Here's how the part is built. I have some questions about the finished solid (model axes, mm). A direction names the side the tool comes from. Coordinates: 2 decimals unless noted, no trailing zeros. Write each loop counter-clockwise with the first axis right and the second up, starting at its lowest first coordinate (ties: lowest second). Pieces come first, ordered by that corner, then holes.
from build123d import *

# Parameters (mm, degrees)
F0_W         = 30
F0_H         = 30
F1_DEPTH     = 30
F2_R         = 5
F3_DEPTH     = 30
F4_R         = 2.5001325449
F5_DEPTH     = 60.001
F6_T1_DEPTH  = 20
F6_T3_DEPTH  = 20
F6_T5_DEPTH  = 20
F6_S9_W      = 5.1
F6_S9_H      = 5.1
F6_T10_DEPTH = 5.1
F6_S15_W     = 5.1
F6_S15_H     = 5.1
F6_T16_DEPTH = 5.1
F6_S21_W     = 5.1
F6_S21_H     = 5.1
F6_T22_DEPTH = 5.1
F6_S27_W     = 5.1
F6_S27_H     = 5.1
F6_T28_DEPTH = 5.1
F6_S33_W     = 5.1
F6_S33_H     = 5.1
F6_T34_DEPTH = 5.1
F6_S39_W     = 5.1
F6_S39_H     = 5.1
F6_T40_DEPTH = 5.1
F6_S45_W     = 5.1
F6_S45_H     = 5.1
F6_T46_DEPTH = 5.1
F6_S51_W     = 5.1
F6_S51_H     = 5.1
F6_T52_DEPTH = 5.1


# Not quite as in the source:
# - a fillet or chamfer that OpenCascade refuses, or shapes differently, is made with other operations: its cross-section is extruded or revolved along the edge and cut away or added


with BuildPart() as f1:
    # F0 (on Front) → F1 (new body)
    with BuildSketch(Plane.XZ):
        Rectangle(F0_W, F0_H)
    extrude(amount=F1_DEPTH)

    # F2 (on face) → F3 (join)
    with BuildSketch(Plane.XZ.offset(30)):
        Circle(F2_R)
    extrude(amount=F3_DEPTH)

    # F4 (on face) → F5 (cut, through all)
    with BuildSketch(Plane.XZ.offset(60)):
        Circle(F4_R)
    extrude(amount=-F5_DEPTH, mode=Mode.SUBTRACT)

    # F6: fillet of radius 5 on 13 edges, made by hand

    # F6_s2 → F6_t1 (cut)
    with BuildSketch(Plane.XZ.offset(5)):
        with BuildLine():
            ThreePointArc((10, 15), (13.5355339059, 13.5355339059), (15, 10))
            Line((15, 10), (15, 15))
            Line((15, 15), (10, 15))
        make_face()
        with BuildLine():
            ThreePointArc((-10, 15), (-13.5355339059, 13.5355339059), (-15, 10))
            Line((-15, 10), (-15, 15))
            Line((-15, 15), (-10, 15))
        make_face()
        with BuildLine():
            ThreePointArc((-15, -10), (-13.5355339059, -13.5355339059), (-10, -15))
            Line((-10, -15), (-15, -15))
            Line((-15, -15), (-15, -10))
        make_face()
        with BuildLine():
            ThreePointArc((15, -10), (13.5355339059, -13.5355339059), (10, -15))
            Line((10, -15), (15, -15))
            Line((15, -15), (15, -10))
        make_face()
    extrude(amount=F6_T1_DEPTH, mode=Mode.SUBTRACT)

    # F6_s4 → F6_t3 (cut)
    with BuildSketch(Plane.YZ.offset(-10)):
        with BuildLine():
            ThreePointArc((-25, 15), (-28.5355339059, 13.5355339059), (-30, 10))
            Line((-30, 10), (-30, 15))
            Line((-30, 15), (-25, 15))
        make_face()
        with BuildLine():
            ThreePointArc((-5, 15), (-1.4644660941, 13.5355339059), (0, 10))
            Line((0, 10), (0, 15))
            Line((0, 15), (-5, 15))
        make_face()
        with BuildLine():
            ThreePointArc((-30, -10), (-28.5355339059, -13.5355339059), (-25, -15))
            Line((-25, -15), (-30, -15))
            Line((-30, -15), (-30, -10))
        make_face()
        with BuildLine():
            ThreePointArc((0, -10), (-1.4644660941, -13.5355339059), (-5, -15))
            Line((-5, -15), (0, -15))
            Line((0, -15), (0, -10))
        make_face()
    extrude(amount=F6_T3_DEPTH, mode=Mode.SUBTRACT)

    # F6_s6 → F6_t5 (cut)
    with BuildSketch(Plane.XY.offset(-10)):
        with BuildLine():
            ThreePointArc((-15, -5), (-13.5355339059, -1.4644660941), (-10, 0))
            Line((-10, 0), (-15, 0))
            Line((-15, 0), (-15, -5))
        make_face()
        with BuildLine():
            ThreePointArc((-15, -25), (-13.5355339059, -28.5355339059), (-10, -30))
            Line((-10, -30), (-15, -30))
            Line((-15, -30), (-15, -25))
        make_face()
        with BuildLine():
            ThreePointArc((15, -5), (13.5355339059, -1.4644660941), (10, 0))
            Line((10, 0), (15, 0))
            Line((15, 0), (15, -5))
        make_face()
        with BuildLine():
            ThreePointArc((15, -25), (13.5355339059, -28.5355339059), (10, -30))
            Line((10, -30), (15, -30))
            Line((15, -30), (15, -25))
        make_face()
    extrude(amount=F6_T5_DEPTH, mode=Mode.SUBTRACT)


with BuildPart() as f6_tool8:
    # F6_s9 → F6_t10 (new body)
    with BuildSketch(Plane.XY.offset(10)):
        with Locations((12.55, -2.45)):
            Rectangle(F6_S9_W, F6_S9_H)
    extrude(amount=F6_T10_DEPTH)

    # F6_s11 → F6_t12 (revolve, cut)
    with BuildSketch(Plane(origin=(10, -5, 10), x_dir=(-0.7071067812, -0.7071067812, 0), z_dir=(-0.7071067812, 0.7071067812, 0))):
        with BuildLine():
            ThreePointArc((0, -5), (5, 0), (0, 5))
            Line((0, 5), (0, -5))
        make_face()
    revolve(axis=Axis((10, -5, 10), (0, 0, 1)), mode=Mode.SUBTRACT)


with BuildPart() as f1_1:
    add(f1.part)

    # F6_t7: cut F6_tool8
    add(f6_tool8.part, mode=Mode.SUBTRACT)


with BuildPart() as f6_tool14:
    # F6_s15 → F6_t16 (new body)
    with BuildSketch(Plane.XY.offset(10)):
        with Locations((12.55, -27.55)):
            Rectangle(F6_S15_W, F6_S15_H)
    extrude(amount=F6_T16_DEPTH)

    # F6_s17 → F6_t18 (revolve, cut)
    with BuildSketch(Plane(origin=(10, -25, 10), x_dir=(-0.7071067812, 0.7071067812, 0), z_dir=(0.7071067812, 0.7071067812, 0))):
        with BuildLine():
            ThreePointArc((0, -5), (5, 0), (0, 5))
            Line((0, 5), (0, -5))
        make_face()
    revolve(axis=Axis((10, -25, 10), (0, 0, 1)), mode=Mode.SUBTRACT)


with BuildPart() as f1_2:
    add(f1_1.part)

    # F6_t13: cut F6_tool14
    add(f6_tool14.part, mode=Mode.SUBTRACT)


with BuildPart() as f6_tool20:
    # F6_s21 → F6_t22 (new body)
    with BuildSketch(Plane.XY.offset(10)):
        with Locations((-12.55, -2.45)):
            Rectangle(F6_S21_W, F6_S21_H)
    extrude(amount=F6_T22_DEPTH)

    # F6_s23 → F6_t24 (revolve, cut)
    with BuildSketch(Plane(origin=(-10, -5, 10), x_dir=(0.7071067812, -0.7071067812, 0), z_dir=(-0.7071067812, -0.7071067812, 0))):
        with BuildLine():
            ThreePointArc((0, -5), (5, 0), (0, 5))
            Line((0, 5), (0, -5))
        make_face()
    revolve(axis=Axis((-10, -5, 10), (0, 0, 1)), mode=Mode.SUBTRACT)


with BuildPart() as f1_3:
    add(f1_2.part)

    # F6_t19: cut F6_tool20
    add(f6_tool20.part, mode=Mode.SUBTRACT)


with BuildPart() as f6_tool26:
    # F6_s27 → F6_t28 (new body)
    with BuildSketch(Plane.XY.offset(10)):
        with Locations((-12.55, -27.55)):
            Rectangle(F6_S27_W, F6_S27_H)
    extrude(amount=F6_T28_DEPTH)

    # F6_s29 → F6_t30 (revolve, cut)
    with BuildSketch(Plane(origin=(-10, -25, 10), x_dir=(0.7071067812, 0.7071067812, 0), z_dir=(0.7071067812, -0.7071067812, 0))):
        with BuildLine():
            ThreePointArc((0, -5), (5, 0), (0, 5))
            Line((0, 5), (0, -5))
        make_face()
    revolve(axis=Axis((-10, -25, 10), (0, 0, 1)), mode=Mode.SUBTRACT)


with BuildPart() as f1_4:
    add(f1_3.part)

    # F6_t25: cut F6_tool26
    add(f6_tool26.part, mode=Mode.SUBTRACT)


with BuildPart() as f6_tool32:
    # F6_s33 → F6_t34 (new body)
    with BuildSketch(Plane.YZ.offset(-10)):
        with Locations((-27.55, -12.55)):
            Rectangle(F6_S33_W, F6_S33_H)
    extrude(amount=-F6_T34_DEPTH)

    # F6_s35 → F6_t36 (revolve, cut)
    with BuildSketch(Plane(origin=(-10, -25, -10), x_dir=(0, 0.7071067812, 0.7071067812), z_dir=(0, -0.7071067812, 0.7071067812))):
        with BuildLine():
            ThreePointArc((0, -5), (5, 0), (0, 5))
            Line((0, 5), (0, -5))
        make_face()
    revolve(axis=Axis((-10, -25, -10), (-1, 0, 0)), mode=Mode.SUBTRACT)


with BuildPart() as f1_5:
    add(f1_4.part)

    # F6_t31: cut F6_tool32
    add(f6_tool32.part, mode=Mode.SUBTRACT)


with BuildPart() as f6_tool38:
    # F6_s39 → F6_t40 (new body)
    with BuildSketch(Plane.YZ.offset(10)):
        with Locations((-27.55, -12.55)):
            Rectangle(F6_S39_W, F6_S39_H)
    extrude(amount=F6_T40_DEPTH)

    # F6_s41 → F6_t42 (revolve, cut)
    with BuildSketch(Plane(origin=(10, -25, -10), x_dir=(0, 0.7071067812, 0.7071067812), z_dir=(0, 0.7071067812, -0.7071067812))):
        with BuildLine():
            ThreePointArc((0, -5), (5, 0), (0, 5))
            Line((0, 5), (0, -5))
        make_face()
    revolve(axis=Axis((10, -25, -10), (1, 0, 0)), mode=Mode.SUBTRACT)


with BuildPart() as f1_6:
    add(f1_5.part)

    # F6_t37: cut F6_tool38
    add(f6_tool38.part, mode=Mode.SUBTRACT)


with BuildPart() as f6_tool44:
    # F6_s45 → F6_t46 (new body)
    with BuildSketch(Plane.YZ.offset(-10)):
        with Locations((-2.45, -12.55)):
            Rectangle(F6_S45_W, F6_S45_H)
    extrude(amount=-F6_T46_DEPTH)

    # F6_s47 → F6_t48 (revolve, cut)
    with BuildSketch(Plane(origin=(-10, -5, -10), x_dir=(0, -0.7071067812, 0.7071067812), z_dir=(0, -0.7071067812, -0.7071067812))):
        with BuildLine():
            ThreePointArc((0, -5), (5, 0), (0, 5))
            Line((0, 5), (0, -5))
        make_face()
    revolve(axis=Axis((-10, -5, -10), (-1, 0, 0)), mode=Mode.SUBTRACT)


with BuildPart() as f1_7:
    add(f1_6.part)

    # F6_t43: cut F6_tool44
    add(f6_tool44.part, mode=Mode.SUBTRACT)


with BuildPart() as f6_tool50:
    # F6_s51 → F6_t52 (new body)
    with BuildSketch(Plane.YZ.offset(10)):
        with Locations((-2.45, -12.55)):
            Rectangle(F6_S51_W, F6_S51_H)
    extrude(amount=F6_T52_DEPTH)

    # F6_s53 → F6_t54 (revolve, cut)
    with BuildSketch(Plane(origin=(10, -5, -10), x_dir=(0, -0.7071067812, 0.7071067812), z_dir=(0, 0.7071067812, 0.7071067812))):
        with BuildLine():
            ThreePointArc((0, -5), (5, 0), (0, 5))
            Line((0, 5), (0, -5))
        make_face()
    revolve(axis=Axis((10, -5, -10), (1, 0, 0)), mode=Mode.SUBTRACT)


with BuildPart() as f1_8:
    add(f1_7.part)

    # F6_t49: cut F6_tool50
    add(f6_tool50.part, mode=Mode.SUBTRACT)

    # F6_s55 → F6_t56 (revolve, cut)
    with BuildSketch(Plane.XY):
        with BuildLine():
            ThreePointArc((2.5001325449, -55.6699495086), (3.1699672637, -58.1698832353), (5, -60))
            Line((5, -60), (2.5001325449, -60))
            Line((2.5001325449, -60), (2.5001325449, -55.6699495086))
        make_face()
    revolve(axis=Axis((0, -60, 0), (0, -1, 0)), mode=Mode.SUBTRACT)


solid = f1_8.part
1. If I drill on line 1 (Z direction, x = 0.25, y = -17.5); line 2 (Z direction, x = 0, y = -41.5); line 3 (Y direction, x = -1.5, z = 5.5), over which ranges is the centre line in solid material (lowest first)?
2. I want a section at C-C (y = -8.5). List the corners of the cut face in (x, z) for me, then the cut area to 3 significant figures.
3. I want a section at D-D (z = -8). List the corners of the cut face in (x, y) for me, then the cut area to 3 significant figures.
4. I want a section at B-B (z = 0). List the corners of the cut face in (x, y) for me.
5. For pin 1 Ø6 at (x, y) = (-9.5, -25.5) entering from +Z; pin 2 Ø10 at (y, z) = (-39.5, -11.5) entering from -X, each with a flat end and sliding along its axis, tell me the tip position at first contact or that it passes through.
6. On a 3-axis mill with a long thin cutter (end or side, diameter ignored), from which of +Z, -Z, +X, -X, +Y, -Y can I reach the whole of each face in a straight line? I mean faces 4 (the face through (-2, -30, 5)), 5 (the face through (13, -15, 14)). Say none if no direction works.
7. Thinking about a two-plate mould opening in X: for faces 1 (the face through (-2, 0, -2)), 2 (the face through (14, -28, 0)), 3 (the face through (-1.84, -28.22, 1.69)), which applies, pulls with the +X half, pulls with the -X half, needs draft (parallel to the pull), parting line crosses it, or undercut?
8. I want a section at A-A (x = 0). List the corners of the cut face in (y, z) for me, then the cut area to 3 significant figures.
Response values:
1. line 1: z = -15 to -2.49, 2.49 to 15
1. line 2: z = -5 to -2.5, 2.5 to 5
1. line 3: y = -30 to 0
2. outline: (-15, -10) arc R5 ccw to (-10, -15) - (10, -15) arc R5 ccw to (15, -10) - (15, 10) arc R5 ccw to (10, 15) - (-10, 15) arc R5 ccw to (-15, 10) - close; hole circle Ø5 at (0, 0)
2. area: 859 mm2
3. outline: (-15, -25) arc R5 ccw to (-10, -30) - (10, -30) arc R5 ccw to (15, -25) - (15, -5) arc R5 ccw to (10, 0) - (-10, 0) arc R5 ccw to (-15, -5) - close
3. area: 879 mm2
4. outline: (-15, -25) arc R5 ccw to (-10, -30) - (-5, -30) - (-5, -60) arc R5 ccw to (-2.5, -55.67) - (-2.5, 0) - (-10, 0) arc R5 ccw to (-15, -5) - close; (2.5, -55.67) arc R5 ccw to (5, -60) - (5, -30) - (10, -30) arc R5 ccw to (15, -25) - (15, -5) arc R5 ccw to (10, 0) - (2.5, 0) - close
5. pin 1: stops at z = 15
5. pin 2: passes through
6. face 4: -Y
6. face 5: +Z, +X, +Y, -Y
7. face 1: needs draft
7. face 2: pulls with the +X half
7. face 3: undercut
8. outline: (-60, -5) - (-30, -5) - (-30, -10) arc R5 ccw to (-25, -15) - (-5, -15) arc R5 ccw to (0, -10) - (0, -2.5) - (-55.67, -2.5) arc R5 ccw to start; (-60, 5) arc R5 ccw to (-55.67, 2.5) - (0, 2.5) - (0, 10) arc R5 ccw to (-5, 15) - (-25, 15) arc R5 ccw to (-30, 10) - (-30, 5) - close
8. area: 872 mm2
